Drawing for the job (mm, zero at the part's lowest x, y, z). A direction names the side the tool comes from. Round coordinates to 2 decimals unless told otherwise and drop trailing zeros. Loops run counter-clockwise (first coordinate to the right, second up) from the corner with the lowest first, then second, coordinate; pieces in that order, holes last. Notation, with made-up numbers: (77, -14.5) -> (135, -14.5) arc R26 ccw to (135, 9.5) -> close; hole circle Ø5 at (78, 50). An arc over 180 degrees is marked (long way). Put each result on its own line as item: value. Start each with the question number.
Item 1: Flat gauge pins, fed straight in: pin 1 Ø0.9 at (x, z) = (10.5, 6) entering from +Y; pin 2 Ø5 at (x, z) = (6, 25) entering from +Y; pin 3 Ø3.5 at (x, z) = (10, 14.5) entering from +Y; pin 4 Ø3.5 at (x, z) = (10, 25) entering from +Y. Where does each tip first touch, or does it go through?
Item 2: Cut at A-A, the plane z = 7. List the corners of the cut face in (x, y), plus the area to 3 significant figures.
Item 3: Drill centre lines: probe 1 along Z at (x, y) = (5.5, 5.25); probe 2 along X at (y, z) = (5, 8); probe 3 along Y at (x, z) = (1.75, 23.5). Where is each one in solid material? Low to high. Write a range as [from, to].
Item 4: Tool access for the marked faces 1, 2 and 3: list every direction of +Z, -Z, +X, -X, +Y, -Y with a clear straight run to the whole face (end or side of a thin tool).
Item 5: Cut at D-D, the plane y = 6.25. List the corners of the cut face in (x, z).
Item 6: Cut at C-C, the plane y = 1.5. List the corners of the cut face in (x, z), plus the area to 3 significant figures.
Item 7: Cut at B-B, the plane x = 7.25. List the corners of the cut face in (y, z), plus the area to 3 significant figures.
Item 8: Pull direction Z, two halves, no side cores. Call the marked faces 4 and 5: +Z half, -Z half, draft (parallel to the pull), parting line (faces both ways), or undercut.
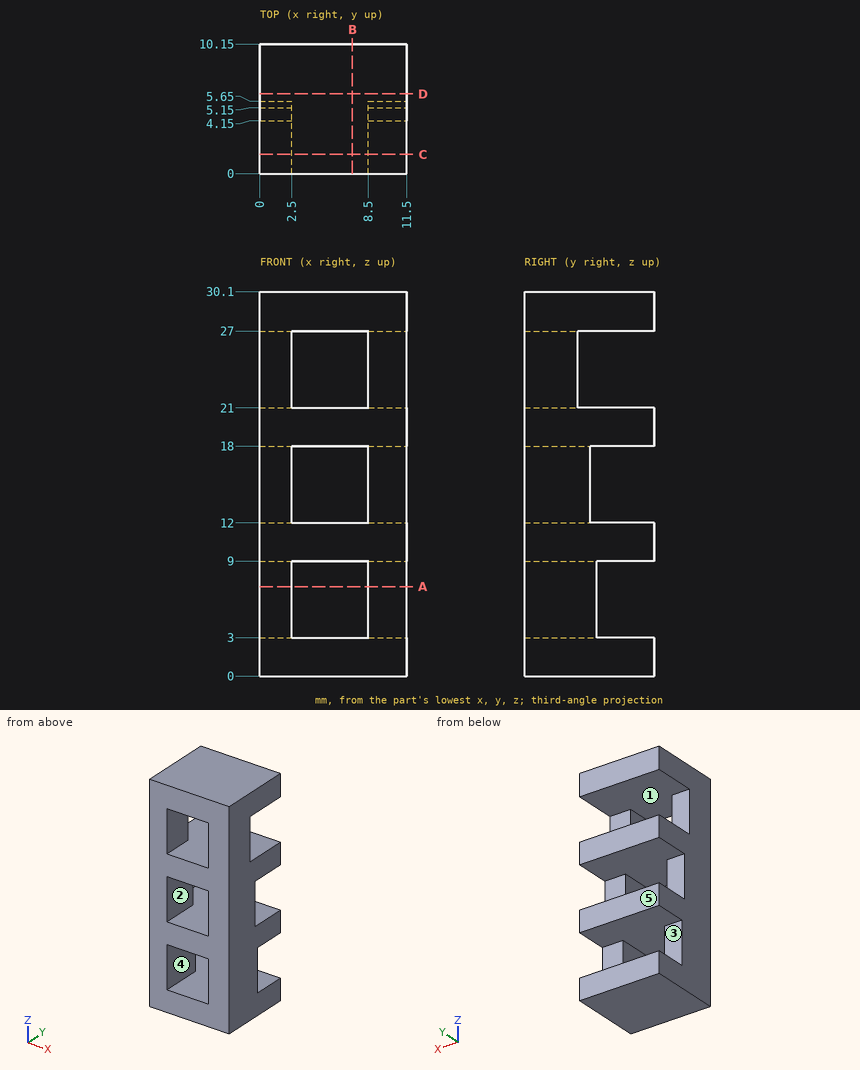
Reply:
1. pin 1: stops at y = 5.65
1. pin 2: stops at y = 10.15
1. pin 3: stops at y = 5.15
1. pin 4: stops at y = 4.15
2. outline: (0, 0) -> (2.5, 0) -> (2.5, 5.65) -> (0, 5.65) -> close; (8.5, 0) -> (11.5, 0) -> (11.5, 5.65) -> (8.5, 5.65) -> close
2. area: 31.1 mm^2
3. probe 1: z = [0, 3], [9, 12], [18, 21], [27, 30.1]
3. probe 2: x = [0, 2.5], [8.5, 11.5]
3. probe 3: y = [0, 4.15]
4. face 1: +Y
4. face 2: +Y, -Y
4. face 3: +X, -X, +Y
5. outline: (0, 0) -> (11.5, 0) -> (11.5, 3) -> (0, 3) -> close; (0, 9) -> (11.5, 9) -> (11.5, 12) -> (0, 12) -> close; (0, 18) -> (11.5, 18) -> (11.5, 21) -> (0, 21) -> close; (0, 27) -> (11.5, 27) -> (11.5, 30.1) -> (0, 30.1) -> close
6. outline: (0, 0) -> (11.5, 0) -> (11.5, 30.1) -> (0, 30.1) -> close; hole (2.5, 3) -> (8.5, 3) -> (8.5, 9) -> (2.5, 9) -> close; hole (2.5, 12) -> (8.5, 12) -> (8.5, 18) -> (2.5, 18) -> close; hole (2.5, 21) -> (8.5, 21) -> (8.5, 27) -> (2.5, 27) -> close
6. area: 238 mm^2
7. outline: (0, 0) -> (10.15, 0) -> (10.15, 3) -> (0, 3) -> close; (0, 9) -> (10.15, 9) -> (10.15, 12) -> (0, 12) -> close; (0, 18) -> (10.15, 18) -> (10.15, 21) -> (0, 21) -> close; (0, 27) -> (10.15, 27) -> (10.15, 30.1) -> (0, 30.1) -> close
7. area: 123 mm^2
8. face 4: undercut
8. face 5: draft
